```python
from build123d import *

# Parameters (mm, degrees)
BOSS_EXTRUDE1_DEPTH = 54.9
FILLET1_R           = 1
SKETCH2_R           = 1.8
CUT_EXTRUDE1_DEPTH  = 200
CUT_EXTRUDE2_DEPTH  = 2
LPATTERN1_COUNT     = 2
LPATTERN1_PITCH     = 38.9


with BuildPart() as part:
    # Sketch1 → Boss-Extrude1 (new body)
    with BuildSketch(Plane.XY):
        Polygon((0, 0), (5.8, 0), (8.7, 3.9), (-2.9, 3.9), align=None)
    extrude(amount=BOSS_EXTRUDE1_DEPTH)

    # Fillet1
    fillet1_edges = [part.edges().sort_by_distance(p)[0] for p in [
        (-2.9, 3.9, 27.45),
        (8.7, 3.9, 27.45),
    ]]
    fillet(fillet1_edges, radius=FILLET1_R)

    # Sketch2 → Cut-Extrude1 (cut)
    with BuildSketch(Plane.XZ):
        with Locations(Location((2.9, 46.9, 0), (0, 0, 270))):
            Circle(SKETCH2_R)
    cut_extrude1 = extrude(amount=-CUT_EXTRUDE1_DEPTH, mode=Mode.SUBTRACT)

    # Sketch3 → Cut-Extrude2 (cut)
    with BuildSketch(Plane.XZ):
        Polygon((2.93968596, 43.551603614), (5.819639312, 45.260170857), (5.779953352, 48.608567243), (2.86031404, 50.248396386), (-0.019639312, 48.539829143), (0.020046648, 45.191432757), align=None)
    cut_extrude2 = extrude(amount=-CUT_EXTRUDE2_DEPTH, mode=Mode.SUBTRACT)

    # LPattern1: Cut-Extrude1, Cut-Extrude2 ×2
    with Locations(*[(0, 0, -i * LPATTERN1_PITCH) for i in range(1, LPATTERN1_COUNT)]):
        add(cut_extrude1, mode=Mode.SUBTRACT)
        add(cut_extrude2, mode=Mode.SUBTRACT)


solid = part.part
```
Here's how the part is built. I have some questions about the finished solid (model axes, mm). A direction names the side the tool comes from. Coordinates: 2 decimals unless noted, no trailing zeros. Order: outer loops, then holes, each group sorted by start corner. A loop starts at its lowest first (then second) coordinate and runs counter-clockwise, first axis right, second up.
Item 1: Which directions (+Z, -Z, +X, -X, +Y, -Y) give clear straight access to the entire face, cutting with the end or side of a thin tool? Please do faces 1 (the face through (1.44, 0.986, 10.506)), 2 (the face through (3, 0, 52)).
Response values:
face 1: -Y
face 2: +Z, -Z, +X, -X, -Y
Item 2: If we section it at D-D, the plane y = 3.35: List the corners of the cut face in (x, z) for me, then the cut area to 3 significant figures.
Response values:
outline: (-1.8, 0) - (7.6, 0) - (7.6, 54.9) - (-1.8, 54.9) - close; hole circle Ø3.6 at (2.9, 8); hole circle Ø3.6 at (2.9, 46.9)
area: 496 mm2
Item 3: If we section it at A-A, the plane z = 40: List the corners of the cut face in (x, y) for me, then the cut area to 3 significant figures.
Response values:
outline: (-1.71, 2.3) - (0, 0) - (5.8, 0) - (7.51, 2.3) arc R1 ccw to (6.71, 3.9) - (-0.91, 3.9) arc R1 ccw to start
area: 32.2 mm2
Item 4: I'm going to push flat-ended pins straight in: pin 1 Ø1 at (y, z) = (2, 13.5) entering from +X; pin 2 Ø1.8 at (x, z) = (2, 46) entering from -Y; pin 3 Ø4 at (x, z) = (2.9, 46.9) entering from +Y. Where does each tip first touch, or does it pass through?
Response values:
pin 1: stops at x = 7.63
pin 2: stops at y = 2
pin 3: stops at y = 3.9
Item 5: If we section it at B-B, the plane y = 1.2: List the corners of the cut face in (x, z) for me.
Response values:
outline: (-0.89, 0) - (6.69, 0) - (6.69, 54.9) - (-0.89, 54.9) - close; hole (-0.02, 9.64) - (0.02, 6.29) - (2.94, 4.65) - (5.82, 6.36) - (5.78, 9.71) - (2.86, 11.35) - close; hole (-0.02, 48.54) - (0.02, 45.19) - (2.94, 43.55) - (5.82, 45.26) - (5.78, 48.61) - (2.86, 50.25) - close
Item 6: If we section it at C-C, the plane x = 4.25: List the corners of the cut face in (y, z) for me, then the cut area to 3 significant figures.
Response values:
outline: (0, 0) - (3.9, 0) - (3.9, 6.81) - (2, 6.81) - (2, 5.43) - (0, 5.43) - close; (0, 10.57) - (2, 10.57) - (2, 9.19) - (3.9, 9.19) - (3.9, 45.71) - (2, 45.71) - (2, 44.33) - (0, 44.33) - close; (0, 49.47) - (2, 49.47) - (2, 48.09) - (3.9, 48.09) - (3.9, 54.9) - (0, 54.9) - close
area: 185 mm2
Item 7: I need wall thicknesses on probe 1 along Z at (x, y) = (3, 2.3); probe 2 along Z at (x, y) = (2.5, 0.25); probe 3 along Y at (x, z) = (1.25, 7). Which ranges of each line are inside material? Lowest first, please.
Response values:
probe 1: z = 0 to 6.2, 9.8 to 45.1, 48.7 to 54.9
probe 2: z = 0 to 4.9, 11.13 to 43.8, 50.03 to 54.9
probe 3: y = 2 to 3.9
Item 8: Thinking about a two-plate mould opening in X: for faces 3 (the face through (3, 0, 3)), 4 (the face through (2, 2, 45)), 5 (the face through (6.644, 1.136, 27.066)), which applies, pulls with the +X half, pulls with the -X half, needs draft (parallel to the pull), parting line crosses it, or undercut?
Response values:
face 3: needs draft
face 4: undercut
face 5: pulls with the +X half
